The model under review builds one solid part; all positions refer to its coordinate system, in mm. Face numbers are marked on the shaded views. A direction names the side the tool comes from. Round coordinates to 2 decimals unless told otherwise and drop trailing zeros. Order: outer loops, then holes, each group sorted by start corner. A loop starts at its lowest first (then second) coordinate and runs counter-clockwise, first axis right, second up. Notation, with made-up numbers: M 67.5,23 L 80.5,23 A25 ccw 80.5,39 Z; hole C -27,37 d11. An arc over 180 degrees is marked long. Answer as a JSON object with one key per item and string values. Group by question number.
1) Consider section B-B, the plane y = 9.75. Write out the cut boundary in (x, z).
2) The part is to be moulded in two halves that separate along Y. For the marked faces 1, 2 and 3, say which applies: +Y half, -Y half, draft (parallel to the pull), parting line (faces both ways), or undercut.
3) For the marked faces 4 and 5, list the 3-axis set-ups (+Z, -Z, +X, -X, +Y, -Y) from which the entire face can be reached by the end or side of a thin tool; tool diameter is ignored.
4) To check wall thickness, follow line 1 (Y direction, x = -0.55, z = -2); line 2 (Z direction, x = -1.25, y = 11.25); line 3 (Y direction, x = -0.5, z = 1.25). State the ranges of each line that lie inside material, in increasing order.
5) Insertion check: pin 1 Ø3 at (x, y) = (-1.5, 8) entering from +Z; pin 2 Ø0.6 at (x, y) = (1.5, 11.5) entering from -Z; pin 3 Ø1.5 at (x, y) = (-1.5, 5.5) entering from -Z. Each pin has a flat end and moves straight along its axis. Give the tip position at first contact, or say it passes through.
6) Consider section A-A, the plane y = 1. Write out the cut boundary in (x, z).
Autodesk Inventor part; units mm, degrees
ref_plane "YZ Plane" through (0, 0, 0) normal (1, 0, 0) x (0, 1, 0)
ref_plane "XZ Plane" through (0, 0, 0) normal (0, 1, 0) x (-1, 0, 0)
ref_plane "XY Plane" through (0, 0, 0) normal (0, 0, 1) x (1, 0, 0)
sketch "Sketch1" plane through (0, 0, 0) normal (0, 0, 1) x (1, 0, 0)
  line L0 (0, 0) -> (-1.5, 1.5)
  line L1 (-1.5, 1.5) -> (-1.5, 9)
  line L2 (-1.5, 9) -> (-1.25, 9)
  line L3 (-1.25, 9) -> (-1.25, 10)
  line L4 (-1.25, 10) -> (-3, 10)
  line L5 (-3, 10) -> (-3, 12)
  line L6 (-3, 12) -> (0, 12)
  line L7 (0, 12) -> (0, 0)
  dimension "d0" = 2
  dimension "d1" = 3
  dimension "d2" = 1.5
  dimension "d3" = 0.25
  dimension "d4" = 1
  dimension "d5" = 12
  dimension "d6" = 45
revolve "Revolution1" add sketch "Sketch1" angle 360 about axis through (0, 12, 0) along (0, -1, 0)
thread "Thread1"
sketch "Sketch2" plane through (0, 12, 0) normal (0, 1, 0) x (1, 0, 0)
  line L0 (5, 0.35) -> (-5, 0.35)
  line L1 (-5, 0.35) -> (-5, -0.35)
  line L2 (-5, -0.35) -> (5, -0.35)
  line L3 (5, -0.35) -> (5, 0.35)
  line L4 (5, 0.35) -> (-5, -0.35) construction
  line L5 (-5, 0.35) -> (5, -0.35) construction
  point P0 (0, 0)
  dimension "d10" = 10
  dimension "d11" = 0.7
fillet "Fillet1" radius 0.25 1 edges at (3, 12, 0)
extrude "Extrusion2" cut sketch "Sketch2" against normal blind 0.7
properties part number "Screw-M3-Fine-GapSet-2" material "Brass, Soft Yellow"
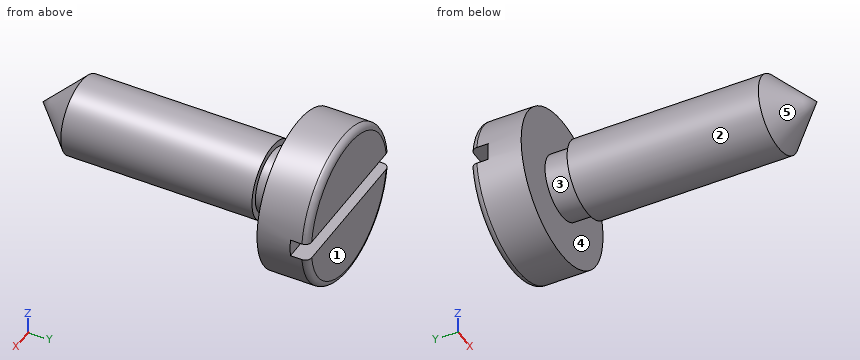
Results list:
{
 "1": {"outline": "C 0,0 d2.5"},
 "2": {"face 1": "+Y half", "face 2": "draft", "face 3": "undercut"},
 "3": {"face 4": "none", "face 5": "-Y"},
 "4": {"line 1": "10 to 12", "line 2": "-2.73 to 2.73", "line 3": "1.35 to 9, 10 to 12"},
 "5": {"pin 1": "z = 1.5", "pin 2": "z = -2.75", "pin 3": "z = -1.3"},
 "6": {"outline": "C 0,0 d2"}
}
